CAD build for the part. Positions are in the model's coordinates, mm. A direction names the side the tool comes from. Round coordinates to 2 decimals unless told otherwise and drop trailing zeros. Write each loop counter-clockwise with the first axis right and the second up, starting at its lowest first coordinate (ties: lowest second). Pieces come first, ordered by that corner, then holes. Notation, with made-up numbers: (41, -19) -> (90, -19) arc R10 cw to (90, -9) -> close; hole circle Ø7 at (2, -39). An arc over 180 degrees is marked (long way). Put each result on its own line as item: value. Start each with the question number.
1. 3-axis set-ups, long thin cutter, end or side, ignore diameter. For faces 1 (the cylindrical face through (-1.5, -0.07, 6.9)), 2 (the flat face through (0, 0, 15.3)), 3 (the flat face through (-8, 0, 15)), 4 (the flat face through (8, 0, 15)): which of +Z, -Z, +X, -X, +Y, -Y reach the whole face in a straight line?
2. Saw through at D-D on x = 0. List the corners of the cut face in (y, z), and give its area (3 significant figures).
3. Saw through at C-C on z = 6. List the corners of the cut face in (x, y), and give its area (3 significant figures).
4. Saw through at A-A on z = 42. List the corners of the cut face in (x, y), and give its area (3 significant figures).
5. Pull direction Y, two halves, no side cores. Call faces 5 (the flat face through (-4, 0, 7)), 6 (the flat face through (0, 0, 14)), 7 (the flat face through (0, -2, 7)): pulls with the +Y half, pulls with the -Y half, needs draft (parallel to the pull), parting line crosses it, or undercut.
6. Flat gauge pin, fed straight in: P1, Ø2, axis at y = -1, z = 5.5, coming from the +X side. Where does the tip first touch, or does it go through?
7. Drill centre lines: line 1 (Y direction, x = 0, z = 9); line 2 (X direction, y = 0, z = 8.25); line 3 (X direction, y = -1.05, z = 21.5). Where is each one in solid material? Low to high. Write a range as from..to.
8. Saw through at B-B on y = 0. List the corners of the cut face in (x, z).
from build123d import *

# Parameters (mm, degrees)
F0_W     = 8
F0_H     = 4
F1_DEPTH = 15
F2_R     = 1.5
F3_DEPTH = 14
F4_W     = 23.7
F4_H     = 4
F5_DEPTH = 0.3
F6_R     = 1
F7_W     = 0.3
F7_H     = 4
F8_DEPTH = 30


with BuildPart() as f1:
    # F0 (on Top) → F1 (new body)
    with BuildSketch(Plane.XY):
        Rectangle(F0_W, F0_H)
    extrude(amount=F1_DEPTH)

    # F2 (on face) → F3 (cut)
    with BuildSketch(Plane(origin=(0, 0, 0), x_dir=(1, 0, 0), z_dir=(0, 0, -1))):
        Circle(F2_R)
    extrude(amount=-F3_DEPTH, mode=Mode.SUBTRACT)

    # F4 (on face) → F5 (join)
    with BuildSketch(Plane.XY.offset(15)):
        Rectangle(F4_W, F4_H)
    extrude(amount=F5_DEPTH)

    # F6
    f6_edges = [f1.edges().sort_by_distance(p)[0] for p in [
        (-4, 0, 15),
        (4, 0, 15),
    ]]
    fillet(f6_edges, radius=F6_R)

    # F7 (on face) → F8 (join)
    with BuildSketch(Plane.XY.offset(15.3)):
        with Locations((-11.7, 0)):
            Rectangle(F7_W, F7_H)
        with Locations((11.7, 0)):
            Rectangle(F7_W, F7_H)
    extrude(amount=F8_DEPTH)


solid = f1.part
Return value:
1. face 1: -Z
1. face 2: +Z, +Y, -Y
1. face 3: -Z, -X, +Y, -Y
1. face 4: -Z, +X, +Y, -Y
2. outline: (-2, 0) -> (-1.5, 0) -> (-1.5, 14) -> (1.5, 14) -> (1.5, 0) -> (2, 0) -> (2, 15.3) -> (-2, 15.3) -> close
2. area: 19.2 mm^2
3. outline: (-4, -2) -> (4, -2) -> (4, 2) -> (-4, 2) -> close; hole circle Ø3 at (0, 0)
3. area: 24.9 mm^2
4. outline: (-11.85, -2) -> (-11.55, -2) -> (-11.55, 2) -> (-11.85, 2) -> close; (11.55, -2) -> (11.85, -2) -> (11.85, 2) -> (11.55, 2) -> close
4. area: 2.40 mm^2
5. face 5: needs draft
5. face 6: undercut
5. face 7: pulls with the -Y half
6. P1: stops at x = 4
7. line 1: y = -2..-1.5, 1.5..2
7. line 2: x = -4..-1.5, 1.5..4
7. line 3: x = -11.85..-11.55, 11.55..11.85
8. outline: (-11.85, 15) -> (-5, 15) arc R1 cw to (-4, 14) -> (-4, 0) -> (-1.5, 0) -> (-1.5, 14) -> (1.5, 14) -> (1.5, 0) -> (4, 0) -> (4, 14) arc R1 cw to (5, 15) -> (11.85, 15) -> (11.85, 45.3) -> (11.55, 45.3) -> (11.55, 15.3) -> (-11.55, 15.3) -> (-11.55, 45.3) -> (-11.85, 45.3) -> close
